Geometry check sheet. Reference: the model listing, model coordinates, mm. A direction names the side the tool comes from. Give positions to 0.01 mm unless a question says otherwise; leave off trailing zeros. Write each loop counter-clockwise with the first axis right and the second up, starting at its lowest first coordinate (ties: lowest second). Pieces come first, ordered by that corner, then holes. Notation, with made-up numbers: (85, 14.5) - (135, 14.5) arc R13 cw to (135, 19.5) - close; hole circle Ø2 at (83, 16). An arc over 180 degrees is marked (long way). Use a Markdown table: item, result.
```python
from build123d import *

# Parameters (mm, degrees)
SKETCH1_W           = 50
SKETCH1_H           = 49.8
SKETCH1_R           = 14
BOSS_EXTRUDE1_DEPTH = 32
SKETCH5_R           = 2
CUT_EXTRUDE2_DEPTH  = 48.634126422
SKETCH12_W          = 30
SKETCH12_H          = 8
BOSS_EXTRUDE3_DEPTH = 18
CUT_EXTRUDE3_DEPTH  = 30
FILLET5_R           = 5
FILLET6_R           = 5
FILLET8_R           = 4
SKETCH14_R          = 2
CUT_EXTRUDE4_DEPTH  = 10
SKETCH16_R          = 2.75
CUT_EXTRUDE5_DEPTH  = 69.330154398
FILLET10_R          = 8
FILLET11_R          = 5


with BuildPart() as part:
    # Sketch1 → Boss-Extrude1 (new body)
    with BuildSketch(Plane.XY):
        Rectangle(SKETCH1_W, SKETCH1_H)
        Circle(SKETCH1_R, mode=Mode.SUBTRACT)
    extrude(amount=BOSS_EXTRUDE1_DEPTH)

    # Sketch5 → Cut-Extrude2 (cut, through all)
    with BuildSketch(Plane.XY.offset(32)):
        with Locations((20, -18.9)):
            Circle(SKETCH5_R)
        with Locations((-20, 19.9)):
            Circle(SKETCH5_R)
    extrude(amount=-CUT_EXTRUDE2_DEPTH, mode=Mode.SUBTRACT)

    # Sketch12 → Boss-Extrude3 (add)
    with BuildSketch(Plane(origin=(0, 0, 25), x_dir=(-1, 0, 0), z_dir=(0, 0, -1))):
        with Locations((-40, 8.9)):
            Rectangle(SKETCH12_W, SKETCH12_H)
    extrude(amount=BOSS_EXTRUDE3_DEPTH)

    # Sketch13 → Cut-Extrude3 (cut)
    with BuildSketch(Plane(origin=(55, 0, 0), x_dir=(0, 0, -1), z_dir=(1, 0, 0))):
        Polygon((-18.550538513, 12.9), (-21.449461487, 12.9), (-20.75, 11.4), (-19.25, 11.4), align=None)
        Polygon((-10.550538513, 12.9), (-13.449461487, 12.9), (-12.75, 11.4), (-11.25, 11.4), align=None)
    extrude(amount=-CUT_EXTRUDE3_DEPTH, mode=Mode.SUBTRACT)

    # Fillet5
    fillet5_edges = [part.edges().sort_by_distance(p)[0] for p in [
        (25, 8.9, 25),
    ]]
    fillet(fillet5_edges, radius=FILLET5_R)

    # Fillet6
    fillet6_edges = [part.edges().sort_by_distance(p)[0] for p in [
        (25, 8.9, 7),
    ]]
    fillet(fillet6_edges, radius=FILLET6_R)

    # Fillet8
    fillet8_edges = [part.edges().sort_by_distance(p)[0] for p in [
        (25, 4.9, 16),
    ]]
    fillet(fillet8_edges, radius=FILLET8_R)

    # Sketch14 → Cut-Extrude4 (cut)
    with BuildSketch(Plane(origin=(0, 12.9, 0), x_dir=(1, 0, 0), z_dir=(0, 1, 0))):
        with Locations(Location((50, -16, 0), (0, 0, 180))):
            Circle(SKETCH14_R)
        with Locations(Location((30.5, -16, 0), (0, 0, 180))):
            Circle(SKETCH14_R)
    extrude(amount=-CUT_EXTRUDE4_DEPTH, mode=Mode.SUBTRACT)

    # Sketch16 → Cut-Extrude5 (cut, through all)
    with BuildSketch(Plane.XY.offset(32)):
        with Locations((0, 19)):
            Circle(SKETCH16_R)
        with Locations((13.435028843, 13.435028843)):
            Circle(SKETCH16_R)
        with Locations((13.435028843, -13.435028843)):
            Circle(SKETCH16_R)
        with Locations((0, -19)):
            Circle(SKETCH16_R)
        with Locations((-13.435028843, -13.435028843)):
            Circle(SKETCH16_R)
        with Locations((-13.435028843, 13.435028843)):
            Circle(SKETCH16_R)
    extrude(amount=-CUT_EXTRUDE5_DEPTH, mode=Mode.SUBTRACT)

    # Fillet10
    # the kernel refuses this fillet: 8 mm, written as the material it takes off along each edge
    with BuildSketch(Plane(origin=(45, -24.9, 32), x_dir=(0, 1, 0), z_dir=(-1, 0, 0)), Plane(origin=(45, -24.9, 0), x_dir=(0, 0, 1), z_dir=(-1, 0, 0)), Plane(origin=(-45, 24.9, 0), x_dir=(0, 0, 1), z_dir=(1, 0, 0))) as fillet10_piece_1:
        with BuildLine():
            CenterArc((FILLET10_R, FILLET10_R), FILLET10_R, 180, 90)
            Line((0, FILLET10_R), (0, 0))
            Line((0, 0), (FILLET10_R, 0))
        make_face()
    extrude(amount=90, mode=Mode.SUBTRACT)
    with BuildSketch(Plane(origin=(-45, 24.9, 32), x_dir=(0, 0, -1), z_dir=(1, 0, 0))) as fillet10_piece_2:
        with BuildLine():
            CenterArc((FILLET10_R, -FILLET10_R), FILLET10_R, 90, 90)
            Line((0, -FILLET10_R), (0, 0))
            Line((0, 0), (FILLET10_R, 0))
        make_face()
    extrude(amount=90, mode=Mode.SUBTRACT)

    # Fillet11
    # the kernel refuses this fillet: 5 mm, written as the material it takes off along each edge
    with BuildSketch(Plane(origin=(25, -24.9, -4.5), x_dir=(0, 1, 0), z_dir=(0, 0, 1))) as fillet11_piece_1:
        with BuildLine():
            CenterArc((FILLET11_R, FILLET11_R), FILLET11_R, 180, 90)
            Line((0, FILLET11_R), (0, 0))
            Line((0, 0), (FILLET11_R, 0))
        make_face()
    extrude(amount=41, mode=Mode.SUBTRACT)
    with BuildSketch(Plane(origin=(25, 24.9, -4.5), x_dir=(0, -1, 0), z_dir=(0, 0, 1))) as fillet11_piece_2:
        with BuildLine():
            CenterArc((FILLET11_R, -FILLET11_R), FILLET11_R, 90, 90)
            Line((0, -FILLET11_R), (0, 0))
            Line((0, 0), (FILLET11_R, 0))
        make_face()
    extrude(amount=41, mode=Mode.SUBTRACT)


solid = part.part
```
1) Section check B-B on x = 0. Record the boundary of the cut face in (y, z), then the cut area to 3 significant figures.
Working result:
| item | result |
|---|---|
| outline | (-24.9, 8) arc R8 ccw to (-21.75, 1.64) - (-21.75, 30.36) arc R8 ccw to (-24.9, 24) - close; (-16.25, 0) - (-14, 0) - (-14, 32) - (-16.25, 32) - close; (14, 0) - (16.25, 0) - (16.25, 32) - (14, 32) - close; (21.75, 1.64) arc R8 ccw to (24.9, 8) - (24.9, 24) arc R8 ccw to (21.75, 30.36) - close |
| area | 301 mm² |
2) Material ranges on L1, parallel to X at y = -20, z = 4.5; L2, parallel to Y at x = -20, z = 15.5; L3, parallel to X at y = -18, z = 4, recorded low to high. Write a range as from..to.
Working result:
| item | result |
|---|---|
| L1 | x = -25..-2.56, 2.56..18.33, 21.67..25 |
| L2 | y = -24.9..17.9, 21.9..24.9 |
| L3 | x = -25..-2.56, 2.56..18.21, 21.79..25 |
3) Mould release check, pull along Y, two halves, no side actions. Record for faces 1 (the flat face through (0, -15, 0)), 2 (the cylindrical face through (12.932, -5.362, 15.776)), 3 (the cylindrical face through (26.141, 3.697, 16.196)), 4 (the cylindrical face through (-0.358, -16.273, 16.224)): pulls with the +Y half, pulls with the -Y half, needs draft (parallel to the pull), parting line crosses it, or undercut.
Working result:
| item | result |
|---|---|
| face 1 | needs draft |
| face 2 | undercut |
| face 3 | pulls with the -Y half |
| face 4 | undercut |
4) Depth check by flat-ended pin: P1, Ø9.5, axis at x = 45, z = 7, coming from the +Y side; P2, Ø10, axis at x = 39, z = 19, coming from the -Y side; P3, Ø1.6, axis at x = 42, z = 20, coming from the +Y side. Enter the tip coordinate at first touch or a pass-through.
Working result:
| item | result |
|---|---|
| P1 | stops at y = 12.9 |
| P2 | stops at y = 4.9 |
| P3 | stops at y = 11.51 |
5) Set-up check for faces 5 (the flat face through (40, 12.9, 16)), 6 (the flat face through (40.21, 12.16, 13.105)), 7 (the flat face through (43, 9, 25)): record each of +Z, -Z, +X, -X, +Y, -Y from which the full face is reachable in a straight line by a thin tool's end or side.
Working result:
| item | result |
|---|---|
| face 5 | +Z, -Z, +X, +Y |
| face 6 | +X, +Y |
| face 7 | +Z, +X, +Y, -Y |
6) Section check C-C on z = 16. Count the separate pieces of the cut face and the enclosed holes in it, then the cut area to 3 significant figures.
Working result:
| item | result |
|---|---|
| separate pieces | 3 |
| enclosed holes | 9 |
| area | 1,880 mm² |
7) Section check A-A on y = 0. Record the boundary of the cut face in (x, z), then the cut area to 3 significant figures.
Working result:
| item | result |
|---|---|
| outline | (-25, 0) - (-14, 0) - (-14, 32) - (-25, 32) - close; (14, 0) - (25, 0) - (25, 32) - (14, 32) - close |
| area | 704 mm² |
